from build123d import *

# Parameters (mm, degrees)
F0_W        = 167.5
F0_H        = 85
F0_W_2      = 2.5
F0_H_2      = 2.5
F0_H_3      = 82.5
F1_DEPTH    = 100
F2_T        = -2.5
F3_W        = 2.5
F3_H        = 167.5
F3_W_2      = 167.5
F3_H_2      = 2.5
F4_DEPTH    = 300
F5_T        = 2.5
F5_T3_DEPTH = 172.5
F5_T5_DEPTH = 172.5
F5_T7_DEPTH = 100
F6_DEPTH    = 50
F7_T        = 2.5
F7_T3_DEPTH = 172.5
F7_T5_DEPTH = 172.5
F7_T7_DEPTH = 100
F7_T9_DEPTH = 302.5


# Not quite as in the source:
# - a shell that OpenCascade refuses in one call is made with other operations: the cavity is built on its own and cut out


with BuildPart() as f1:
    # F0 (on Top) → F1 (new body)
    with BuildSketch(Plane.XY):
        Polygon((82.5, -85), (85, -85), (85, 82.5), (82.5, 82.5), (82.5, 0), align=None)
        with Locations((-1.25, -42.5)):
            Rectangle(F0_W, F0_H)
        with Locations((83.75, 83.75)):
            Rectangle(F0_W_2, F0_H_2)
        with Locations((-1.25, 41.25)):
            Rectangle(F0_W, F0_H_3)
        with Locations((-1.25, 83.75)):
            Rectangle(F0_W, F0_H_2)
    extrude(amount=F1_DEPTH)

    # F2
    f2_openings = [f1.faces().sort_by_distance(p)[0] for p in [
        (85, 0, 50),
        (0, -85, 50),
    ]]
    offset(amount=F2_T, openings=f2_openings)

    # F3 (on face) → F4 (join)
    with BuildSketch(Plane.XY.offset(100)):
        with Locations((-83.75, -1.25)):
            Rectangle(F3_W, F3_H)
        with Locations((1.25, -1.25)):
            Rectangle(F3_W_2, F3_H)
        with Locations((-83.75, 83.75)):
            Rectangle(F3_W, F3_H_2)
        with Locations((1.25, 83.75)):
            Rectangle(F3_W_2, F3_H_2)
    extrude(amount=F4_DEPTH)

    # F5: shell of thickness 2.5, made by hand


with BuildPart() as f5_core1:
    # F5_t2: copy of F1
    add(f1.part)

    # the walls: a layer under each face that stays
    f5_faces = [f5_core1.faces().sort_by_distance(p)[0] for p in [
        (0, 85, 200),
        (0, 0, 0),
        (1.25, -1.25, 2.5),
        (1.25, 82.5, 50),
        (-82.5, -1.25, 50),
        (1.25, -1.25, 97.5),
        (-85, 0, 200),
        (0, 0, 400),
    ]]
    thicken(f5_faces, amount=-F5_T, mode=Mode.SUBTRACT)

    # F5_s4 → F5_t3 (cut)
    with BuildSketch(Plane.YZ.offset(-85)):
        Polygon((82.475, 2.525), (82.5, 0), (85, 0), (85, 2.5), align=None)
        Polygon((82.475, 97.475), (85, 97.5), (85, 100), (82.5, 100), align=None)
    extrude(amount=F5_T3_DEPTH, mode=Mode.SUBTRACT)

    # F5_s6 → F5_t5 (cut)
    with BuildSketch(Plane.XZ.offset(-85)):
        Polygon((-82.475, 2.525), (-82.5, 0), (-85, 0), (-85, 2.5), align=None)
        Polygon((-82.475, 97.475), (-85, 97.5), (-85, 100), (-82.5, 100), align=None)
    extrude(amount=F5_T5_DEPTH, mode=Mode.SUBTRACT)

    # F5_s8 → F5_t7 (cut)
    with BuildSketch(Plane.XY):
        Polygon((-82.475, 82.475), (-82.5, 85), (-85, 85), (-85, 82.5), align=None)
    extrude(amount=F5_T7_DEPTH, mode=Mode.SUBTRACT)


with BuildPart() as f1_1:
    add(f1.part)

    # what is left inside the walls is the cavity
    f5_cavity = [f5_core1.part.solids().sort_by_distance(p)[0] for p in [
        (1.25, 82.475, 298.333333),
    ]]
    add(f5_cavity, mode=Mode.SUBTRACT)

    # F6 (add): a face of the model
    f6_faces = [f1_1.faces().sort_by_distance(p)[0] for p in [
        (0, 0, 400),
    ]]
    extrude(f6_faces, amount=F6_DEPTH)

    # F7: shell of thickness 2.5, made by hand


with BuildPart() as f7_core1:
    # F7_t2: copy of F1
    add(f1_1.part)

    # the walls: a layer under each face that stays
    f7_faces = [f7_core1.faces().sort_by_distance(p)[0] for p in [
        (0, 85, 225),
        (0, 0, 0),
        (1.25, -1.25, 2.5),
        (1.25, 82.5, 50),
        (-82.5, -1.25, 50),
        (1.25, -1.25, 97.5),
        (1.25, -1.25, 100),
        (1.25, 82.5, 248.75),
        (-82.5, -1.25, 248.75),
        (1.25, -1.25, 397.5),
        (-85, 0, 225),
        (0, 0, 450),
    ]]
    thicken(f7_faces, amount=-F7_T, mode=Mode.SUBTRACT)

    # F7_s4 → F7_t3 (cut)
    with BuildSketch(Plane.YZ.offset(-85)):
        Polygon((82.475, 2.525), (82.5, 0), (85, 0), (85, 2.5), align=None)
        Polygon((82.475, 97.475), (85, 97.5), (85, 100), (82.5, 100), align=None)
        Polygon((82.475, 100.025), (82.5, 97.5), (85, 97.5), (85, 100), align=None)
        Polygon((82.475, 397.475), (85, 397.5), (85, 400), (82.5, 400), align=None)
    extrude(amount=F7_T3_DEPTH, mode=Mode.SUBTRACT)

    # F7_s6 → F7_t5 (cut)
    with BuildSketch(Plane.XZ.offset(-85)):
        Polygon((-82.475, 2.525), (-82.5, 0), (-85, 0), (-85, 2.5), align=None)
        Polygon((-82.475, 97.475), (-85, 97.5), (-85, 100), (-82.5, 100), align=None)
        Polygon((-82.475, 100.025), (-82.5, 97.5), (-85, 97.5), (-85, 100), align=None)
        Polygon((-82.475, 397.475), (-85, 397.5), (-85, 400), (-82.5, 400), align=None)
    extrude(amount=F7_T5_DEPTH, mode=Mode.SUBTRACT)

    # F7_s8 → F7_t7 (cut)
    with BuildSketch(Plane.XY):
        Polygon((-82.475, 82.475), (-82.5, 85), (-85, 85), (-85, 82.5), align=None)
    extrude(amount=F7_T7_DEPTH, mode=Mode.SUBTRACT)

    # F7_s10 → F7_t9 (cut)
    with BuildSketch(Plane.XY.offset(97.5)):
        Polygon((-82.475, 82.475), (-82.5, 85), (-85, 85), (-85, 82.5), align=None)
    extrude(amount=F7_T9_DEPTH, mode=Mode.SUBTRACT)


with BuildPart() as f1_2:
    add(f1_1.part)

    # what is left inside the walls is the cavity
    f7_cavity = [f7_core1.part.solids().sort_by_distance(p)[0] for p in [
        (1.25, -29.166667, 447.475),
    ]]
    add(f7_cavity, mode=Mode.SUBTRACT)


solid = f1_2.part
Geometry check sheet. Reference: the model listing, model coordinates, mm. A direction names the side the tool comes from. Give positions to 0.01 mm unless a question says otherwise; leave off trailing zeros. Loops run counter-clockwise (first coordinate to the right, second up) from the corner with the lowest first, then second, coordinate; pieces in that order, holes last.
(1) Depth check by flat-ended pin: pin 1 Ø2 at (y, z) = (15, 231) entering from +X; pin 2 Ø1 at (x, z) = (-38, 258) entering from -Y. Enter the tip coordinate at first touch or a pass-through.
From the geometry:
pin 1: stops at x = -82.5
pin 2: stops at y = 82.5
(2) Section check A-A on y = -35. Record the cut outline in (x, z), then the cut area to 3 significant figures.
From the geometry:
outline: (-85, 0) - (85, 0) - (85, 2.5) - (-82.5, 2.5) - (-82.5, 97.5) - (85, 97.5) - (85, 100) - (-82.5, 100) - (-82.5, 397.5) - (85, 397.5) - (85, 400) - (-82.5, 400) - (-82.5, 447.5) - (85, 447.5) - (85, 450) - (-85, 450) - close
area: 2,800 mm2
(3) Section check C-C on z = 133. Record the cut outline in (x, y), then the cut area to 3 significant figures.
From the geometry:
outline: (-85, -85) - (-82.5, -85) - (-82.5, 82.5) - (85, 82.5) - (85, 85) - (-85, 85) - close
area: 844 mm2
(4) Thickness scan on L1, parallel to Z at x = 53, y = -50; L2, parallel to Y at x = 16.5, z = 338.5; L3, parallel to X at y = -33, z = 159.5. Record the ranges inside material, lowest first.
From the geometry:
L1: z = 0 to 2.5, 97.5 to 100, 397.5 to 400, 447.5 to 450
L2: y = 82.5 to 85
L3: x = -85 to -82.5
(5) Set-up check for faces 4 (the flat face through (2, 82.5, 247)), 5 (the flat face through (-85, 1, 222)): record each of +Z, -Z, +X, -X, +Y, -Y from which the full face is reachable in a straight line by a thin tool's end or side.
From the geometry:
face 4: +X, -Y
face 5: +Z, -Z, -X, +Y, -Y
(6) Section check B-B on x = 18. Record the cut outline in (y, z).
From the geometry:
outline: (-85, 0) - (85, 0) - (85, 450) - (-85, 450) - (-85, 447.5) - (82.5, 447.5) - (82.5, 400) - (-85, 400) - (-85, 397.5) - (82.5, 397.5) - (82.5, 100) - (-85, 100) - (-85, 97.5) - (82.5, 97.5) - (82.5, 2.5) - (-85, 2.5) - close
(7) Release check for a two-part mould opening along Z. For faces 1 (the flat face through (-1, 1, 0)), 2 (the flat face through (0, 0, 400)), 3 (the flat face through (1, 85, 222)) record: released by +Z, released by -Z, zero draft, split by the parting line, or undercut.
From the geometry:
face 1: released by -Z
face 2: undercut
face 3: zero draft
